Geometry check sheet. Reference: the model listing, model coordinates, mm. A direction names the side the tool comes from. Round coordinates to 2 decimals unless told otherwise and drop trailing zeros. Order: outer loops, then holes, each group sorted by start corner. A loop starts at its lowest first (then second) coordinate and runs counter-clockwise, first axis right, second up.
(1) Go/stop test with flat-tipped pins: pin 1 (1.3 mm diameter, centred on x = -7.5, y = 1, fed in from +Z); pin 2 (2 mm diameter, centred on y = 3, z = 3.5, fed in from -X); pin 3 (1 mm diameter, centred on y = -2, z = 0.5, fed in from +X). Record where each tip stops, or that it passes through.
(2) Sectioned sample at D-D (z = 3.7). Record the boundary of the cut face in (x, y), plus the area to 3 significant figures.
(3) Sectioned sample at C-C (z = 0.65). Record the boundary of the cut face in (x, y), plus the area to 3 significant figures.
(4) Material ranges on line 1 along Z through (x, y) = (-6.25, 3); line 2 along X through (y, z) = (-0.25, 1.4); line 3 along X through (y, z) = (-1.75, 2.1), recorded low to high.
(5) Sectioned sample at A-A (z = 2.65). Record the boundary of the cut face in (x, y), plus the area to 3 significant figures.
(6) Set-up check for faces 1 (the face through (-9, 0, 2)), 2 (the face through (6.5, 0.1, 4)), 3 (the face through (-7, 0, 3)): record each of +Z, -Z, +X, -X, +Y, -Y from which the full face is reachable in a straight line by a thin tool's end or side.
(7) Sectioned sample at B-B (x = -4.25). Record the boundary of the cut face in (y, z).
Autodesk Fusion 360 part; units mm, degrees
sketch "Twist-Lock2 lock" plane through (0, 0, 0) normal (0, 0, 1) x (1, 0, 0)
  line L0 (7.7942, -4.5) -> (-7.7942, -4.5)
  line L1 (-7.7942, 4.5) -> (7.7942, 4.5)
  arc A0 (-7.7942, 4.5) -> (-7.7942, -4.5) centre (0, 0) ccw
  arc A1 (7.7942, -4.5) -> (7.7942, 4.5) centre (0, 0) ccw
  arc A2 (-4.6904, 4.5) -> (-4.6904, -4.5) centre (0, 0) ccw
  arc A3 (4.6904, -4.5) -> (4.6904, 4.5) centre (0, 0) ccw
sketch "Twist-Lock2 hole" plane through (0, 0, 0) normal (0, 0, 1) x (1, 0, 0)
  arc A0 (-8.093, 3.9375) -> (-8.093, -3.9375) centre (0, 0) ccw
  arc A1 (8.093, -3.9375) -> (8.093, 3.9375) centre (0, 0) ccw
  arc A2 (4.4192, 4.7667) -> (-4.4192, 4.7667) centre (0, 0) ccw
  arc A3 (-4.4192, -4.7667) -> (4.4192, -4.7667) centre (0, 0) ccw
  line L0 (7.1937, 4.5) -> (5.099, 4.5)
  line L1 (-5.099, 4.5) -> (-7.1937, 4.5)
  line L2 (-7.1937, -4.5) -> (-5.099, -4.5)
  line L3 (5.099, -4.5) -> (7.1937, -4.5)
  arc A4 (-5.099, 4.5) -> (-4.4192, 4.7667) centre (-5.099, 5.5) ccw
  arc A5 (-7.1937, 4.5) -> (-8.093, 3.9375) centre (-7.1937, 3.5) ccw
  arc A6 (-8.093, -3.9375) -> (-7.1937, -4.5) centre (-7.1937, -3.5) ccw
  arc A7 (-4.4192, -4.7667) -> (-5.099, -4.5) centre (-5.099, -5.5) ccw
  arc A8 (5.099, -4.5) -> (4.4192, -4.7667) centre (5.099, -5.5) ccw
  arc A9 (7.1937, -4.5) -> (8.093, -3.9375) centre (7.1937, -3.5) ccw
  arc A10 (8.093, 3.9375) -> (7.1937, 4.5) centre (7.1937, 3.5) ccw
  arc A11 (4.4192, 4.7667) -> (5.099, 4.5) centre (5.099, 5.5) ccw
  dimension "d26" = 1
extrude "Extrude1" add sketch "Twist-Lock2 lock" along normal blind 3
extrude "Extrude2" add sketch "Twist-Lock2 lock" along normal blind 5 contours L0 L1 A2 A3
fillet "Fillet1" radius 1.1 4 edges at (7.7942, -4.5, 1.5) (-7.7942, -4.5, 1.5) (-7.7942, 4.5, 1.5) (7.7942, 4.5, 1.5)
chamfer "Chamfer1" distance 1 angle 45 8 edges at (-7.718, -4.3303, 0) (-9, 0, 0) (-7.718, 4.3303, 0) (0, 4.5, 0) (7.718, 4.3303, 0) (9, 0, 0) (7.718, -4.3303, 0) (0, -4.5, 0)
equation "Plate_thickness = 2 mm"
equation "Lock_thickness = 3 mm"
equation "d7 = Lock_thickness"
equation "d9 = Lock_thickness + Plate_thickness"
Answer below:
1. pin 1: stops at z = 3
1. pin 2: stops at x = -8.74
1. pin 3: stops at x = 8.79
2. outline: (-4.69, -4.5) - (4.69, -4.5) arc R6.5 ccw to (4.69, 4.5) - (-4.69, 4.5) arc R6.5 ccw to start
2. area: 107 mm2
3. outline: (-7.81, -3.72) arc R0.75 ccw to (-7.13, -4.15) - (7.13, -4.15) arc R0.75 ccw to (7.81, -3.72) arc R8.65 ccw to (7.81, 3.72) arc R0.75 ccw to (7.13, 4.15) - (-7.13, 4.15) arc R0.75 ccw to (-7.81, 3.72) arc R8.65 ccw to start
3. area: 138 mm2
4. line 1: z = 0 to 3
4. line 2: x = -9 to 9
4. line 3: x = -8.83 to 8.83
5. outline: (-8.12, -3.87) arc R1.1 ccw to (-7.13, -4.5) - (7.13, -4.5) arc R1.1 ccw to (8.12, -3.87) arc R9 ccw to (8.12, 3.87) arc R1.1 ccw to (7.13, 4.5) - (-7.13, 4.5) arc R1.1 ccw to (-8.12, 3.87) arc R9 ccw to start
5. area: 155 mm2
6. face 1: +Z, -Z, -X
6. face 2: +Z, +X
6. face 3: +Z, -X
7. outline: (-4.5, 1) - (-3.5, 0) - (3.5, 0) - (4.5, 1) - (4.5, 5) - (-4.5, 5) - close
